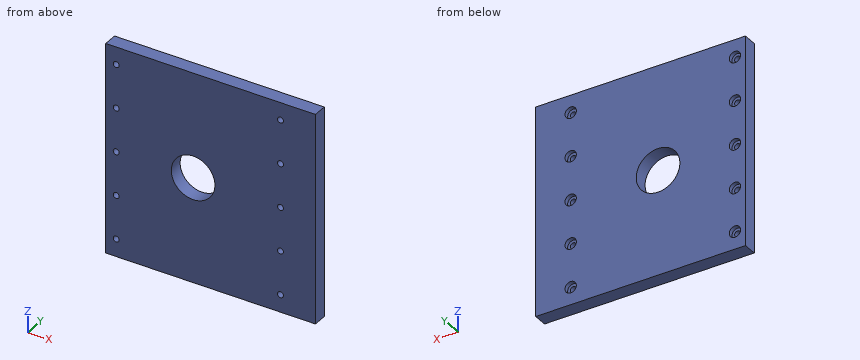
from build123d import *

# Parameters (mm, degrees)
SKETCH1_W                                            = 120
SKETCH1_H                                            = 120
BOSS_EXTRUDE1_DEPTH                                  = 8
CBORE_FOR_M3_HEX_SOCKET_THIN_HEAD_CAP_SC_D           = 3.4
CBORE_FOR_M3_HEX_SOCKET_THIN_HEAD_CAP_SC_CBORE_D     = 6.5
CBORE_FOR_M3_HEX_SOCKET_THIN_HEAD_CAP_SC_CBORE_DEPTH = 2.4
F_25_0MM_DOWEL_HOLE1_D                               = 25
F_25_0MM_DOWEL_HOLE1_DEPTH                           = 10
F_25_0MM_DOWEL_HOLE1_TIP                             = 7.510757738


with BuildPart() as part:
    # Sketch1 → Boss-Extrude1 (new body)
    with BuildSketch(Plane(origin=(0, 0, 0), x_dir=(1, 0, 0), z_dir=(0, 1, 0))):
        with Locations((60, 60)):
            Rectangle(SKETCH1_W, SKETCH1_H)
    extrude(amount=BOSS_EXTRUDE1_DEPTH)

    # CBORE for M3 Hex Socket Thin Head Cap Screw1 (through all)
    with Locations(Plane(origin=(0, 8, 0), x_dir=(1, 0, 0), z_dir=(0, 1, 0))):
        with Locations((100, 110), (6, 110), (6, 85), (6, 60), (6, 35), (6, 10), (100, 60), (100, 35), (100, 10), (100, 85)):
            CounterBoreHole(CBORE_FOR_M3_HEX_SOCKET_THIN_HEAD_CAP_SC_D / 2, CBORE_FOR_M3_HEX_SOCKET_THIN_HEAD_CAP_SC_CBORE_D / 2, CBORE_FOR_M3_HEX_SOCKET_THIN_HEAD_CAP_SC_CBORE_DEPTH)

    # Ø25.0mm Dowel Hole1
    with Locations(Plane(origin=(0, 8, 0), x_dir=(1, 0, 0), z_dir=(0, 1, 0))):
        with Locations((50, 60)):
            Hole(F_25_0MM_DOWEL_HOLE1_D / 2, depth=F_25_0MM_DOWEL_HOLE1_DEPTH)
            with Locations((0, 0, -(F_25_0MM_DOWEL_HOLE1_DEPTH + F_25_0MM_DOWEL_HOLE1_TIP / 2))):  # 118° drill point
                Cone(0, F_25_0MM_DOWEL_HOLE1_D / 2, F_25_0MM_DOWEL_HOLE1_TIP, mode=Mode.SUBTRACT)


solid = part.part
Here's how the part is built. I have some questions about the finished solid (model axes, mm). Coordinates: 2 decimals unless noted, no trailing zeros. Write each loop counter-clockwise with the first axis right and the second up, starting at its lowest first coordinate (ties: lowest second). Pieces come first, ordered by that corner, then holes.
1) I'm going to push a flat-ended pin straight in: pin 1 (6 mm diameter, centred on x = 6, z = -60, fed in from +Y). Where does the tip first touch, or does it pass through?
Filled in:
pin 1: stops at y = 5.6
2) If we section it at C-C (y = 2.5): Count the separate pieces of the cut face and the enclosed holes in it, plus the area to 3 significant figures.
Filled in:
separate pieces: 1
enclosed holes: 11
area: 13,800 mm2
3) If we section it at A-A (x = 50): List the corners of the cut face in (y, z) for me.
Filled in:
outline: (0, -120) - (8, -120) - (8, -72.5) - (0, -72.5) - close; (0, -47.5) - (8, -47.5) - (8, 0) - (0, 0) - close
4) If we section it at B-B (z = -35): List the corners of the cut face in (x, y) for me.
Filled in:
outline: (0, 0) - (4.3, 0) - (4.3, 5.6) - (2.75, 5.6) - (2.75, 8) - (0, 8) - close; (7.7, 0) - (98.3, 0) - (98.3, 5.6) - (96.75, 5.6) - (96.75, 8) - (9.25, 8) - (9.25, 5.6) - (7.7, 5.6) - close; (101.7, 0) - (120, 0) - (120, 8) - (103.25, 8) - (103.25, 5.6) - (101.7, 5.6) - close
5) If I drill on line 1 (Z direction, x = 6, y = 3.35); line 2 (Z direction, x = 6, y = 7.4); line 3 (X direction, y = 4.3, z = -110), over which ranges is the centre line in solid material (lowest first)?
Filled in:
line 1: z = -120 to -111.7, -108.3 to -86.7, -83.3 to -61.7, -58.3 to -36.7, -33.3 to -11.7, -8.3 to 0
line 2: z = -120 to -113.25, -106.75 to -88.25, -81.75 to -63.25, -56.75 to -38.25, -31.75 to -13.25, -6.75 to 0
line 3: x = 0 to 4.3, 7.7 to 98.3, 101.7 to 120
